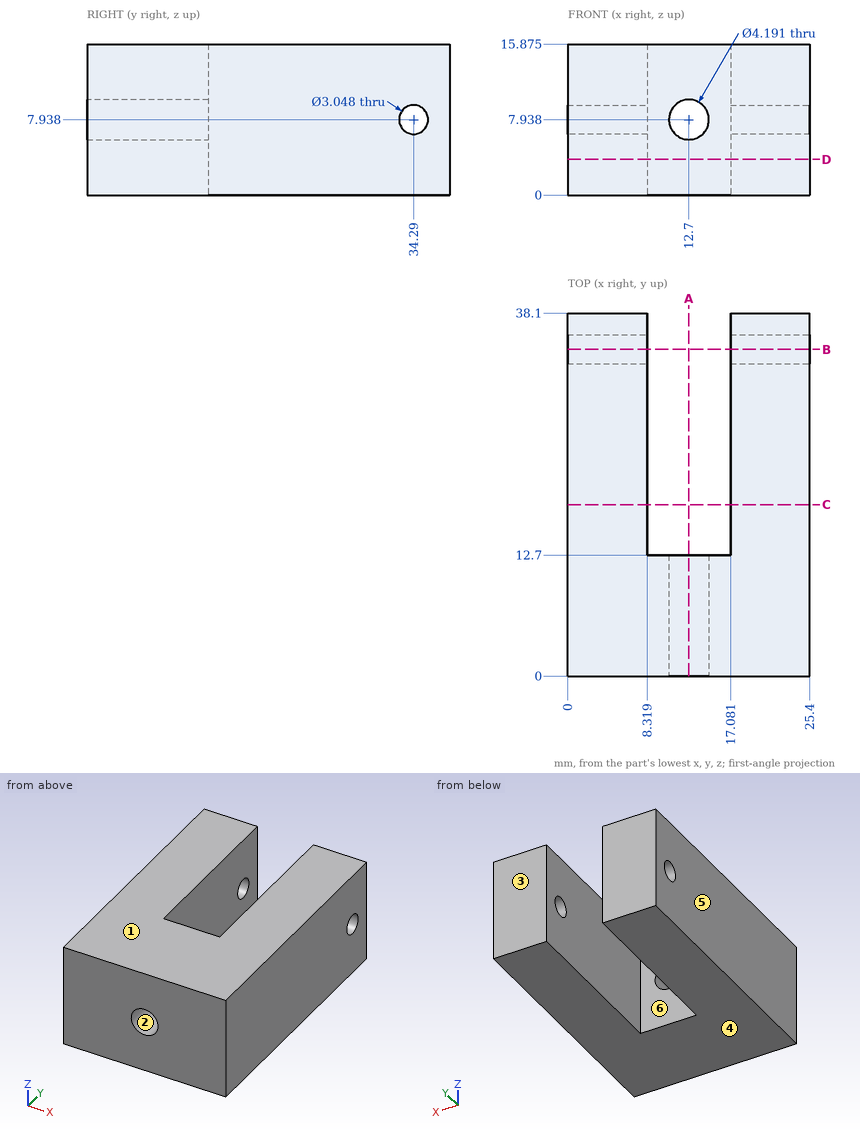
Input: dimensioned drawing with shaded views. Units: mm. Origin: part minimum x, y, z. A direction names the side the tool comes from. Round coordinates to 2 decimals unless told otherwise and drop trailing zeros. Loops run counter-clockwise (first coordinate to the right, second up) from the corner with the lowest first, then second, coordinate; pieces in that order, holes last. Notation, with made-up numbers: (37, -6) -> (88, -6) arc R33 ccw to (88, 32) -> close; hole circle Ø9 at (17.5, -0.75). An arc over 180 degrees is marked (long way). One line per item, written item: value.
(1) Set-up query: the marked faces 5 and 6. Return all of +Z, -Z, +X, -X, +Y, -Y with unobstructed straight access to the full face (end or side cutting, diameter ignored); none if empty.
Geometry check:
face 5: +Z, -Z, -X, +Y, -Y
face 6: +Z, -Z, +Y
(2) Section A-A (x = 12.7). Return the cut outline in (y, z) (1 decimal), plus the area to 3 significant figures.
Geometry check:
outline: (0, 0) -> (12.7, 0) -> (12.7, 5.8) -> (0, 5.8) -> close; (0, 10) -> (12.7, 10) -> (12.7, 15.9) -> (0, 15.9) -> close
area: 148 mm2
(3) Section D-D (z = 3.75). Return the cut outline in (x, y), plus the area to 3 significant figures.
Geometry check:
outline: (0, 0) -> (25.4, 0) -> (25.4, 38.1) -> (17.08, 38.1) -> (17.08, 12.7) -> (8.32, 12.7) -> (8.32, 38.1) -> (0, 38.1) -> close
area: 745 mm2
(4) Material intervals for line 1 (X direction, y = 25, z = 2.25); line 2 (Y direction, x = 17, z = 12.5); line 3 (Y direction, x = 21.5, z = 9) (1 decimal), sorted ascending. Write a range as [from, to].
Geometry check:
line 1: [0, 8.32], [17.08, 25.4]
line 2: [0, 12.7]
line 3: [0, 33.2], [35.4, 38.1]
(5) Mould query, pull axis Z, two halves, no side actions, for the marked faces 1, 2, 3 and 4. Classes: pulls with the +Z half, pulls with the -Z half, needs draft (parallel to the pull), parting line crosses it, or undercut.
Geometry check:
face 1: pulls with the +Z half
face 2: undercut
face 3: needs draft
face 4: pulls with the -Z half
(6) Section C-C (y = 18). Return the cut outline in (x, z) (1 decimal).
Geometry check:
outline: (0, 0) -> (8.3, 0) -> (8.3, 15.9) -> (0, 15.9) -> close; (17.1, 0) -> (25.4, 0) -> (25.4, 15.9) -> (17.1, 15.9) -> close
(7) Section B-B (y = 34.29). Return the cut outline in (x, z) (1 decimal).
Geometry check:
outline: (0, 0) -> (8.3, 0) -> (8.3, 6.4) -> (0, 6.4) -> close; (0, 9.5) -> (8.3, 9.5) -> (8.3, 15.9) -> (0, 15.9) -> close; (17.1, 0) -> (25.4, 0) -> (25.4, 6.4) -> (17.1, 6.4) -> close; (17.1, 9.5) -> (25.4, 9.5) -> (25.4, 15.9) -> (17.1, 15.9) -> close
(8) Pin query (flat end, axial travel): pin 1 (6.5 mm diameter, centred on x = 12.7, z = 7.94, fed in from +Y); pin 2 (1.8 mm diameter, centred on y = 34.29, z = 7.94, fed in from -X). Return the tip coordinate at first contact, or that it passes through.
Geometry check:
pin 1: y = 12.7
pin 2: through
